from build123d import *

# Parameters (mm, degrees)
CYLINDER150_R       = 1.7
CYLINDER150_DEPTH   = 11
CYLINDER151_R       = 1.7
CYLINDER151_DEPTH   = 11
CYLINDER157_R       = 2.25
CYLINDER157_DEPTH   = 8
CYLINDER156_R       = 1
CYLINDER156_DEPTH   = 5
CYLINDER147_R       = 1
CYLINDER147_DEPTH   = 1
ARRAY_COUNT         = 3
BOX_W               = 3
BOX_H               = 8
BOX_DEPTH           = 5
CYLINDER153_R       = 11
CYLINDER153_DEPTH   = 5
BOX001_W            = 3
BOX001_H            = 8
BOX001_DEPTH        = 5
CYLINDER158_R       = 4
CYLINDER158_DEPTH   = 5
CYLINDER_R          = 4
CYLINDER_DEPTH      = 5
CUT_PLACEMENT_ANGLE = 180
BOX008_W            = 2
BOX008_H            = 9.2
BOX008_DEPTH        = 6
CYLINDER198_R       = 11.6
CYLINDER198_DEPTH   = 6
CYLINDER199_R       = 4.6
CYLINDER199_DEPTH   = 6
CYLINDER200_R       = 4.6
CYLINDER200_DEPTH   = 6
BOX009_W            = 2
BOX009_H            = 9.2
BOX009_DEPTH        = 6


with BuildPart() as obj1:
    # Cylinder150 → Cylinder150 (new body)
    with BuildSketch(Plane(origin=(-13, 0, 0), x_dir=(1, 0, 0), z_dir=(0, 0, 1))):
        Circle(CYLINDER150_R)
    extrude(amount=CYLINDER150_DEPTH)


with BuildPart() as obj2:
    # Cylinder151 → Cylinder151 (new body)
    with BuildSketch(Plane(origin=(13, 0, 0), x_dir=(1, 0, 0), z_dir=(0, 0, 1))):
        Circle(CYLINDER151_R)
    extrude(amount=CYLINDER151_DEPTH)


with BuildPart() as sealsubtraction:
    # Cylinder157 → Cylinder157 (new body)
    with BuildSketch(Plane.XY.offset(2.5)):
        Circle(CYLINDER157_R)
    extrude(amount=CYLINDER157_DEPTH)


with BuildPart() as bottomwireoutlet:
    # Cylinder156 → Cylinder156 (new body)
    with BuildSketch(Plane.XY.offset(-2)):
        Circle(CYLINDER156_R)
    extrude(amount=CYLINDER156_DEPTH)


with BuildPart() as fusion013:
    # Cylinder147 → Cylinder147 (new body)
    with BuildSketch(Plane.XY.offset(4.5)):
        Circle(CYLINDER147_R)
    extrude(amount=CYLINDER147_DEPTH)

    # Fusion: union SealSubtraction, BottomWireOutlet
    add(sealsubtraction.part)
    add(bottomwireoutlet.part)


with BuildPart() as fusion013_1:
    # Fusion placement: moved
    add(fusion013.part.moved(Location((4.25, 0, 0))))

    # Array: Fusion013 ×3 about axis
    array_axis = Axis((0, 0, 0), (0, 0, 1))


with BuildPart() as fusion013_2:
    add(fusion013_1.part)
    for i in range(1, ARRAY_COUNT):
        add(fusion013_1.part.rotate(array_axis, i * 360 / ARRAY_COUNT))

    # Fusion013: union obj1, obj2
    add(obj1.part)
    add(obj2.part)


with BuildPart() as mountcube1:
    # Box → Box (new body)
    with BuildSketch(Plane(origin=(-13, -4, 0), x_dir=(1, 0, 0), z_dir=(0, 0, 1))):
        with Locations((1.5, 4)):
            Rectangle(BOX_W, BOX_H)
    extrude(amount=BOX_DEPTH)


with BuildPart() as body:
    # Cylinder153 → Cylinder153 (new body)
    with BuildSketch(Plane.XY):
        Circle(CYLINDER153_R)
    extrude(amount=CYLINDER153_DEPTH)


with BuildPart() as mountcube002:
    # Box001 → Box001 (new body)
    with BuildSketch(Plane(origin=(10, -4, 0), x_dir=(1, 0, 0), z_dir=(0, 0, 1))):
        with Locations((1.5, 4)):
            Rectangle(BOX001_W, BOX001_H)
    extrude(amount=BOX001_DEPTH)


with BuildPart() as mountflange002:
    # Cylinder158 → Cylinder158 (new body)
    with BuildSketch(Plane(origin=(13, 0, 0), x_dir=(1, 0, 0), z_dir=(0, 0, 1))):
        Circle(CYLINDER158_R)
    extrude(amount=CYLINDER158_DEPTH)


with BuildPart() as cut:
    # Cylinder → Cylinder (new body)
    with BuildSketch(Plane(origin=(-13, 0, 0), x_dir=(1, 0, 0), z_dir=(0, 0, 1))):
        Circle(CYLINDER_R)
    extrude(amount=CYLINDER_DEPTH)

    # Fusion012: union MountCube1, Body, MountCube002, MountFlange002
    add(mountcube1.part)
    add(body.part)
    add(mountcube002.part)
    add(mountflange002.part)

    # Cut: cut Fusion013
    add(fusion013_2.part, mode=Mode.SUBTRACT)


with BuildPart() as cut_1:
    # Cut placement: moved
    add(cut.part.moved(Location((0, 0, 6))).rotate(Axis((0, 0, 6), (1, 0, 0)), CUT_PLACEMENT_ANGLE))


with BuildPart() as cube:
    # Box008 → Box008 (new body)
    with BuildSketch(Plane(origin=(-12, -4.6, 0), x_dir=(1, 0, 0), z_dir=(0, 0, 1))):
        with Locations((1, 4.6)):
            Rectangle(BOX008_W, BOX008_H)
    extrude(amount=BOX008_DEPTH)


with BuildPart() as cylinder:
    # Cylinder198 → Cylinder198 (new body)
    with BuildSketch(Plane.XY):
        Circle(CYLINDER198_R)
    extrude(amount=CYLINDER198_DEPTH)


with BuildPart() as cylinder016:
    # Cylinder199 → Cylinder199 (new body)
    with BuildSketch(Plane(origin=(-13, 0, 0), x_dir=(1, 0, 0), z_dir=(0, 0, 1))):
        Circle(CYLINDER199_R)
    extrude(amount=CYLINDER199_DEPTH)


with BuildPart() as cylinder017:
    # Cylinder200 → Cylinder200 (new body)
    with BuildSketch(Plane(origin=(13, 0, 0), x_dir=(1, 0, 0), z_dir=(0, 0, 1))):
        Circle(CYLINDER200_R)
    extrude(amount=CYLINDER200_DEPTH)


with BuildPart() as cut027:
    # Box009 → Box009 (new body)
    with BuildSketch(Plane(origin=(10, -4.6, 0), x_dir=(1, 0, 0), z_dir=(0, 0, 1))):
        with Locations((1, 4.6)):
            Rectangle(BOX009_W, BOX009_H)
    extrude(amount=BOX009_DEPTH)

    # Fusion014: union Cube, Cylinder, Cylinder016, Cylinder017
    add(cube.part)
    add(cylinder.part)
    add(cylinder016.part)
    add(cylinder017.part)

    # Cut027: cut Cut
    add(cut_1.part, mode=Mode.SUBTRACT)


solid = cut027.part
Model file for the job. Use its own axes, mm. A direction names the side the tool comes from. Round coordinates to 2 decimals unless told otherwise and drop trailing zeros. Loops run counter-clockwise (first coordinate to the right, second up) from the corner with the lowest first, then second, coordinate; pieces in that order, holes last. Notation, with made-up numbers: (27, 31.25) -> (41, 31.25) arc R11 ccw to (41, 38.25) -> close; hole circle Ø1 at (65, 20.25). An arc over 180 degrees is marked (long way). Answer as CSV lines item,"result". Start each with the question number.
1) Slice it at C-C (x = 2.5). List the corners of the cut face in (y, z), plus the area to 3 significant figures.
2) Pin check, flat tips, straight feed: P1, Ø0.8, axis at x = -11.5, z = 4, coming from the -Y side; P2, Ø3, axis at y = -4, z = 2, coming from the -X side; P3, Ø0.8, axis at x = -11, z = 3.5, coming from the +Y side. Stop position of each tip, or through.
3) Slice it at B-B (y = 0). List the corners of the cut face in (x, z), plus the area to 4 significant figures.
4) Slice it at D-D (y = 7.25). List the corners of the cut face in (x, z).
5) Slice it at A-A (z = 0.5). List the corners of the cut face in (x, y).
6) Probe line 1 along Y through (x, z) = (11, 5.25); line 2 along X through (y, z) = (-3, 4.75); line 3 along Y through (x, z) = (-11.5, 4.5). List the from-to ranges inside material, lowest first.
7) Tool access for faces 1 (the face through (-11, -4.6, 3)), 2 (the face through (6.396, -0.676, 2.268)), 3 (the face through (4, 0, 6)): list every direction of +Z, -Z, +X, -X, +Y, -Y with a clear straight run to the whole face (end or side of a thin tool).
8) Mould opens along X. For faces 4 (the face through (11, 4.6, 3)), 5 (the face through (-0.2, -11.6, 3)), 6 (the face through (12, -4, 4)) say: +X half, -X half, draft (parallel to the pull), parting line (faces both ways), or undercut.
Filled in:
1,outline,"(-11.33, 0) -> (11.33, 0) -> (11.33, 6) -> (10.71, 6) -> (10.71, 1) -> (1.41, 1) -> (1.41, 3.5) -> (-1.41, 3.5) -> (-1.41, 1) -> (-10.71, 1) -> (-10.71, 6) -> (-11.33, 6) -> close"
1,area,"35.9 mm2"
2,P1,"stops at y = -4.6"
2,P2,"stops at x = -16.86"
2,P3,"stops at y = 4.71"
3,outline,"(-17.6, 0) -> (17.6, 0) -> (17.6, 6) -> (17, 6) -> (17, 1) -> (14.7, 1) -> (14.7, 6) -> (11.3, 6) -> (11.3, 1) -> (6.5, 1) -> (6.5, 3.5) -> (5.25, 3.5) -> (5.25, 6) -> (3.25, 6) -> (3.25, 3.5) -> (2, 3.5) -> (2, 1) -> (-11.3, 1) -> (-11.3, 6) -> (-14.7, 6) -> (-14.7, 1) -> (-17, 1) -> (-17, 6) -> (-17.6, 6) -> close"
3,area,"91.45 mm2"
4,outline,"(-9.06, 0) -> (9.06, 0) -> (9.06, 6) -> (8.27, 6) -> (8.27, 1) -> (-8.27, 1) -> (-8.27, 6) -> (-9.06, 6) -> close"
5,outline,"(-12, -4.6) -> (-10.65, -4.6) arc R11.6 ccw to (10.65, -4.6) -> (12, -4.6) -> (12, -4.49) arc R4.6 ccw (long way) to (12, 4.49) -> (12, 4.6) -> (10.65, 4.6) arc R11.6 ccw to (-10.65, 4.6) -> (-12, 4.6) -> (-12, 4.49) arc R4.6 ccw (long way) to (-12, -4.49) -> close"
6,line 1,"y = -4.6 to -4, 4 to 4.6"
6,line 2,"x = -16.49 to -15.65, -2.86 to -1.39, 15.65 to 16.49"
6,line 3,"y = -4.6 to -4, -0.8 to 0.8, 4 to 4.6"
7,face 1,"+Z, -Z, -X, -Y"
7,face 2,"+Z"
7,face 3,"+Z, +X, -X, +Y, -Y"
8,face 4,"draft"
8,face 5,"parting line"
8,face 6,"undercut"
